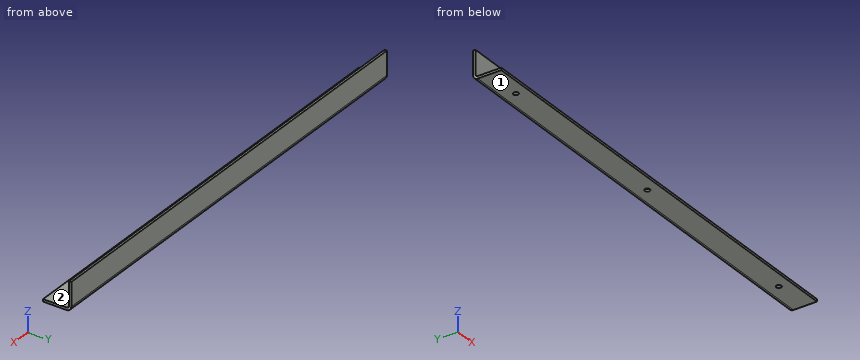
```python
from build123d import *

# Parameters (mm, degrees)
BOSS_EXTRUDE1_DEPTH = 609.6
FILLET1_R           = 3.175
FILLET2_R           = 6.35
SKETCH3_R           = 3.3782
CUT_EXTRUDE1_DEPTH  = 4.175


with BuildPart() as part:
    # Sketch2 → Boss-Extrude1 (new body)
    with BuildSketch(Plane(origin=(0, 0, 0), x_dir=(0, 0, -1), z_dir=(1, 0, 0))):
        Polygon((-38.1, 0), (0, 0), (0, -38.1), (-3.175, -38.1), (-3.175, -3.175), (-38.1, -3.175), align=None)
    extrude(amount=BOSS_EXTRUDE1_DEPTH)

    # Fillet1
    fillet1_edges = [part.edges().sort_by_distance(p)[0] for p in [
        (304.8, -3.175, 3.175),
    ]]
    fillet(fillet1_edges, radius=FILLET1_R)

    # Fillet2
    fillet2_edges = [part.edges().sort_by_distance(p)[0] for p in [
        (304.8, 0, 0),
    ]]
    fillet(fillet2_edges, radius=FILLET2_R)

    # Sketch3 → Cut-Extrude1 (cut, through all)
    with BuildSketch(Plane.XY.offset(3.175)):
        with Locations((304.8, -22.225)):
            Circle(SKETCH3_R)
        with Locations((558.8, -22.225)):
            Circle(SKETCH3_R)
        with Locations((50.8, -22.225)):
            Circle(SKETCH3_R)
    extrude(amount=-CUT_EXTRUDE1_DEPTH, mode=Mode.SUBTRACT)


solid = part.part
```
Geometry check sheet. Reference: the model listing, model coordinates, mm. Face numbers are marked on the shaded views. A direction names the side the tool comes from. Coordinates: 2 decimals unless noted, no trailing zeros. Order: outer loops, then holes, each group sorted by start corner. A loop starts at its lowest first (then second) coordinate and runs counter-clockwise, first axis right, second up.
Q1. Sectioned sample at A-A on x = 479.5. Record the cut outline in (y, z) (3 decimals), and give its area (3 significant figures).
Reply:
outline: (-38.1, 0) - (-6.35, 0) arc R6.35 ccw to (0, 6.35) - (0, 38.1) - (-3.175, 38.1) - (-3.175, 6.35) arc R3.175 cw to (-6.35, 3.175) - (-38.1, 3.175) - close
area: 225 mm2
Q2. Tool access check on the marked faces 1 and 2. Record the directions out of +Z, -Z, +X, -X, +Y, -Y that give a thin tool (end or side, any length) a straight path to the whole face; none if there is none.
Reply:
face 1: -Z, +X, -X, +Y, -Y
face 2: +Z, +X, -X, -Y
Q3. Thickness scan on probe 1 along Y at (x, z) = (50.8, 0.8); probe 2 along Z at (x, y) = (305.5, -28.5) (3 decimals); probe 3 along Y at (x, z) = (366.5, 23) (3 decimals). Record the ranges inside material, lowest first.
Reply:
probe 1: y = -38.1 to -25.6, -18.85 to -3.26
probe 2: z = 0 to 3.175
probe 3: y = -3.175 to 0
Q4. Depth check by flat-ended pin: pin 1 Ø16 at (x, z) = (443, 24.5) entering from -Y (3 decimals); pin 2 Ø8 at (x, y) = (50.8, -22.225) entering from +Z (3 decimals); pin 3 Ø12 at (x, y) = (443, -11) entering from +Z. Enter the tip coordinate at first touch or a pass-through.
Reply:
pin 1: stops at y = -3.175
pin 2: stops at z = 3.175
pin 3: stops at z = 3.48
Q5. Sectioned sample at B-B on y = -31. Record the cut outline in (x, z) (3 decimals).
Reply:
outline: (0, 0) - (609.6, 0) - (609.6, 3.175) - (0, 3.175) - close
Q6. Sectioned sample at C-C on z = 21.5. Record the cut outline in (x, y) (3 decimals).
Reply:
outline: (0, -3.175) - (609.6, -3.175) - (609.6, 0) - (0, 0) - close
